Geometry: final body of the model. Coordinates: model frame, mm. Face numbers are marked on the shaded views. A direction names the side the tool comes from. Give positions to 0.01 mm unless a question says otherwise; leave off trailing zeros. Order: outer loops, then holes, each group sorted by start corner. A loop starts at its lowest first (then second) coordinate and runs counter-clockwise, first axis right, second up. Notation, with made-up numbers: (61, -24.75) - (98, -24.75) arc R20 cw to (98, -0.75) - close; hole circle Ø4 at (4.5, 2.25). An arc over 180 degrees is marked (long way). One line per item, written item: value.
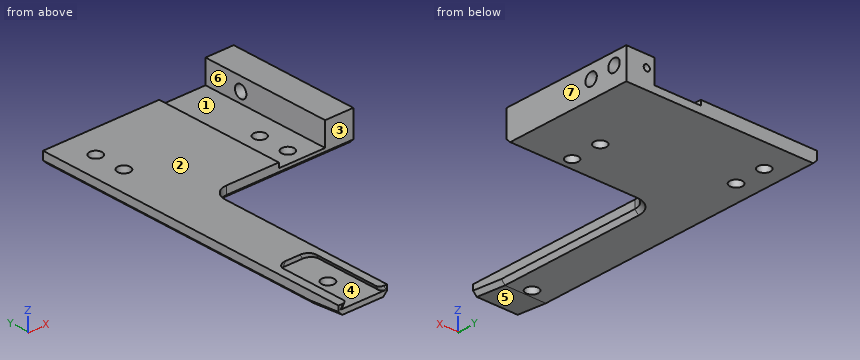
Autodesk Fusion 360 part; units mm, degrees
sketch "Sketch1" plane through (0, 0, 0) normal (0, 1, 0) x (1, 0, 0)
  line L0 (-12.4, 0.775) -> (12.4, 0.775)
  line L1 (12.4, 0.775) -> (12.4, -0.775)
  line L2 (12.4, -0.775) -> (-12.4, -0.775)
  line L3 (-12.4, -0.775) -> (-12.4, 0.775)
  line L4 (-12.4, 0.775) -> (12.4, -0.775) construction
  line L5 (12.4, 0.775) -> (-12.4, -0.775) construction
  dimension "d1" = 24.8
  dimension "d2" = 1.55
extrude "Extrude1" add sketch "Sketch1" along normal mid plane 17
sketch "Sketch4" plane through (0, 8.5, 0) normal (0, 1, 0) x (-1, 0, 0)
  line L0 (12.4, -0.775) -> (12.4, 0.775)
  line L1 (12.4, 0.775) -> (-12.4, 0.775)
  line L2 (-12.4, 0.775) -> (-12.4, -0.775)
  line L3 (-12.4, -0.775) -> (12.4, -0.775)
  line L4 (7.0918, 0.775) -> (6.7692, 0.2162)
  line L5 (6.7692, 0.2162) -> (11.6308, 0.2162)
  line L6 (11.6308, 0.2162) -> (11.3082, 0.775)
  point P0 (9.2, 0.2162)
  dimension "d11" = 60
  dimension "d12" = 60
  dimension "d13" = 4.2164
  dimension "d14" = 0.5588
  dimension "d47" = 3.2
extrude "Extrude3" cut sketch "Sketch4" against normal up to surface (17 mm away) contours L1 L4 L5 L6
sketch "Sketch2" plane through (0, 8.5, 0) normal (0, 1, 0) x (-1, 0, 0)
  line L0 (7.0918, 0.775) -> (-12.4, 0.775)
  line L1 (-12.4, 0.775) -> (-12.4, -0.775)
  line L2 (-12.4, -0.775) -> (12.4, -0.775)
  line L3 (12.4, -0.775) -> (12.4, 0.775)
  line L4 (-2.7118, 0.141) -> (-8.7318, 0.141)
  line L5 (-8.7318, 0.141) -> (-8.7318, 0.775)
  line L6 (-8.7318, 0.775) -> (-2.7118, 0.775)
  line L7 (-2.7118, 0.775) -> (-2.7118, 0.141)
  line L8 (6.7692, 0.2162) -> (7.0918, 0.775)
  line L9 (12.4, 0.775) -> (11.3082, 0.775)
  line L10 (11.3082, 0.775) -> (11.6308, 0.2162)
  line L11 (11.6308, 0.2162) -> (6.7692, 0.2162)
  dimension "d5" = 6.02
  dimension "d6" = 0.634
  dimension "d50" = 9.481
extrude "Extrude2" cut sketch "Sketch2" against normal up to surface (17 mm away) contours L0 L4 L5 L6 L7
sketch "Sketch6" plane through (0, 0, -0.775) normal (0, 0, -1) x (-1, 0, 0)
  line L0 (5.6836, 7) -> (5.6836, -7)
  line L1 (5.6836, -7) -> (6.75, -7)
  line L2 (6.75, -7) -> (6.75, 7)
  line L3 (6.75, 7) -> (5.6836, 7)
  line L4 (-0.15, 7) -> (-6.25, 7)
  line L5 (-5.7218, -6.5) -> (-5.7218, -2.5)
  line L6 (12.4, -8.5) -> (12.4, 8.5)
  line L7 (12.4, 8.5) -> (-12.4, 8.5)
  line L8 (-12.4, 8.5) -> (-12.4, -8.5)
  line L9 (-12.4, -8.5) -> (12.4, -8.5)
  curve L10
  line L11 (-2.7118, -8.5) -> (-8.7318, -8.5)
  line L12 (-8.7318, -8.5) -> (-8.7318, 8.5)
  line L13 (-8.7318, 8.5) -> (-2.7118, 8.5)
  line L14 (-2.7118, 8.5) -> (-2.7118, -8.5)
  point P0 (-5.7218, 7)
  point P1 (-5.7218, -2.5)
  point P2 (-5.7218, -6.5)
  point P3 (6.75, 0)
  point P4 (-5.7218, -4.5)
  point P5 (-5.7218, -8.5)
  point P6 (-5.7218, -8.5)
  dimension "d22" = 4
  dimension "d51" = 2
hole "Hole2" at (5.7218, -2.5, -0.775) at (5.7218, -6.5, -0.775) direction (0, 0, 1) diameter 1.6 depth 3.517 tip angle 118
sketch "Sketch7" plane through (0, 0, -0.775) normal (0, 0, -1) x (-1, 0, 0)
  line L0 (5.6836, 7) -> (5.6836, -7)
  line L1 (5.6836, -7) -> (6.75, -7)
  line L2 (6.75, -7) -> (6.75, 7)
  line L3 (6.75, 7) -> (5.6836, 7)
  line L4 (-6.25, -7) -> (-0.15, -7)
  circle A0 centre (-5.7218, -2.5) radius 0.8
  circle A1 centre (-5.7218, -6.5) radius 0.8
  line L5 (12.4, -8.5) -> (12.4, 8.5)
  line L6 (12.4, 8.5) -> (-12.4, 8.5)
  line L7 (-12.4, 8.5) -> (-12.4, -8.5)
  line L8 (-12.4, -8.5) -> (12.4, -8.5)
  point P0 (-3.2, -7)
  point P1 (-3.2, -4.5)
  dimension "d26" = 2.5
hole "Hole3" [suppressed]
extrude "Extrude4" add 1 faces at (11.1773, -2.8333, 0.775) along direction (0, 0, 1) blind 2.4
sketch "Sketch10" plane through (12.4, 0, 0) normal (1, 0, 0) x (0, 1, 0)
  line L0 (-8.5, -0.775) -> (8.5, -0.775)
  line L1 (8.5, -0.775) -> (8.5, 3.175)
  line L2 (8.5, 3.175) -> (-8.5, 3.175)
  line L3 (-8.5, 3.175) -> (-8.5, -0.775)
  point P0 (3.5, 1.475)
  dimension "d54" = 2.25
  dimension "d59" = 12
hole "Hole6" at (12.4, 3.5, 1.475) direction (-1, 0, 0) diameter 1.623 depth 6.5 tip angle 118
sketch "Sketch11" plane through (0, 8.5, 0) normal (0, 1, 0) x (-1, 0, 0)
  line L0 (11.6308, 0.2162) -> (6.7692, 0.2162)
  line L1 (7.0918, 0.775) -> (-2.7118, 0.775)
  line L2 (-2.7118, 0.775) -> (-2.7118, 0.141)
  line L3 (-2.7118, 0.141) -> (-8.7318, 0.141)
  line L4 (-8.7318, 0.141) -> (-8.7318, 3.175)
  line L5 (-8.7318, 3.175) -> (-12.4, 3.175)
  line L6 (-12.4, 3.175) -> (-12.4, -0.775)
  line L7 (-12.4, -0.775) -> (12.4, -0.775)
  line L8 (12.4, -0.775) -> (12.4, 0.775)
  line L9 (12.4, 0.775) -> (11.3082, 0.775)
  line L10 (11.3082, 0.775) -> (11.6308, 0.2162)
  line L11 (6.7692, 0.2162) -> (7.0918, 0.775)
  point P0 (-9.7318, 1.675)
  dimension "d60" = 1.5
  dimension "d61" = 1
hole "Hole7" at (9.7318, 8.5, 1.675) direction (0, -1, 0) diameter 0.8 depth 3 tip angle 118
sketch "Sketch12" plane through (12.4, 0, 0) normal (1, 0, 0) x (0, 1, 0)
  circle A0 centre (3.5, 1.475) radius 0.8115
  line L0 (-8.5, -0.775) -> (8.5, -0.775)
  line L1 (8.5, -0.775) -> (8.5, 3.175)
  line L2 (8.5, 3.175) -> (-8.5, 3.175)
  line L3 (-8.5, 3.175) -> (-8.5, -0.775)
  line L4 (8.5, 2.075) -> (8.5, 1.275)
  line L5 (5.5, 2.075) -> (5.5, 1.275)
  point P0 (6.75, 1.675)
  point P1 (8.5, 1.675)
  dimension "d66" = 1.75
hole "Hole8" at (12.4, 6.75, 1.675) direction (-1, 0, 0) diameter 1.623 depth 2.6 tip angle 118
fillet "Fillet1" [suppressed]
sketch "Sketch13" plane through (0, -8.5, 0) normal (0, -1, 0) x (1, 0, 0)
  line L0 (8.7318, 3.175) -> (8.7318, 0.141)
  line L1 (8.7318, 0.141) -> (2.7118, 0.141)
  line L2 (2.7118, 0.141) -> (2.7118, 0.775)
  line L3 (2.7118, 0.775) -> (-7.0918, 0.775)
  line L4 (-7.0918, 0.775) -> (-6.7692, 0.2162)
  line L5 (-6.7692, 0.2162) -> (-11.6308, 0.2162)
  line L6 (-11.6308, 0.2162) -> (-11.3082, 0.775)
  line L7 (-11.3082, 0.775) -> (-12.4, 0.775)
  line L8 (-12.4, 0.775) -> (-12.4, -0.775)
  line L9 (-12.4, -0.775) -> (12.4, -0.775)
  line L10 (12.4, -0.775) -> (12.4, 3.175)
  line L11 (12.4, 3.175) -> (8.7318, 3.175)
  line L12 (2.7118, 0.141) -> (2.7118, -0.775)
  line L13 (-6.0918, 0.775) -> (-6.0918, -0.775)
  dimension "d78" = 1
extrude "Extrude5" add sketch "Sketch13" along normal blind 25 contours L3 L4 L5 L6 L7 L8 L9 L13
sketch "Sketch5" plane through (0, 0, -0.775) normal (0, 0, -1) x (1, 0, 0)
  line L0 (-12.4, -8.5) -> (12.4, -8.5)
  line L1 (12.4, -8.5) -> (12.4, 8.5)
  line L2 (12.4, 8.5) -> (-6.0918, 8.5)
  line L3 (-12.4, 33.5) -> (-12.4, -8.5)
  circle A0 centre (5.7218, 2.5) radius 0.8
  circle A1 centre (5.7218, 6.5) radius 0.8
  line L4 (-6.0918, 33.5) -> (-12.4, 33.5)
  line L5 (-6.7692, 33.5) -> (-11.6308, 33.5)
  line L6 (-6.0918, 8.5) -> (-6.0918, 33.5)
  point P0 (-9.2, 33.5)
  point P1 (-9.2, 28.5)
  dimension "d72" = 5
hole "Hole1" at (-9.2, -28.5, -0.775) direction (0, 0, 1) diameter 1.623 end through all
sketch "Sketch14" plane through (-6.0918, 0, 0) normal (1, 0, 0) x (0, 1, 0)
  line L0 (-8.5, 0.243) -> (8.5, 0.243)
  line L1 (8.5, 0.243) -> (8.5, 0.875)
  line L2 (8.5, 0.875) -> (-8.5, 0.875)
  line L3 (-8.5, 0.875) -> (-8.5, 0.243)
  line L4 (-33.5, -0.425) -> (-29.5, -0.775)
  line L5 (-8.5, -0.775) -> (-8.5, 0.775)
  line L6 (-8.5, 0.775) -> (-33.5, 0.775)
  line L7 (-33.5, 0.775) -> (-33.5, -0.775)
  line L8 (-33.5, -0.775) -> (-8.5, -0.775)
  dimension "d88" = 4
  dimension "d89" = 0.35
extrude "Extrude6" cut sketch "Sketch14" against normal through all contours L4 L7 L8
fillet "Fillet2" radius 0.5 2 edges at (-11.4695, -33.5, 0.4956) (-6.9305, -33.5, 0.4956)
sketch "Sketch15" plane through (0, 8.5, 0) normal (0, 1, 0) x (-1, 0, 0)
  circle A0 centre (-9.7318, 1.675) radius 0.4
  line L0 (-8.7318, 0.141) -> (-8.7318, 3.175)
  line L1 (-8.7318, 3.175) -> (-12.4, 3.175)
  line L2 (-12.4, 3.175) -> (-12.4, -0.775)
  line L3 (-12.4, -0.775) -> (12.4, -0.775)
  line L4 (12.4, -0.775) -> (12.4, 0.775)
  line L5 (12.4, 0.775) -> (11.3082, 0.775)
  line L6 (11.3082, 0.775) -> (11.6308, 0.2162)
  line L7 (11.6308, 0.2162) -> (6.7692, 0.2162)
  line L8 (6.7692, 0.2162) -> (7.0918, 0.775)
  line L9 (7.0918, 0.775) -> (-2.7118, 0.775)
  line L10 (-2.7118, 0.775) -> (-2.7118, 0.141)
  line L11 (-2.7118, 0.141) -> (-8.7318, 0.141)
  line L12 (7.0918, 0.775) -> (11.3082, 0.775)
extrude "Extrude7" add sketch "Sketch15" against normal blind 32 contours L6 L7 L8 L12
sketch "Sketch16" plane through (0, 0, 0.775) normal (0, 0, 1) x (-1, 0, 0)
  ellipse E0 centre (11.8856, 33) end of major axis (11.3082, 33) minor radius 0.5 (11.8856, 33.5) -> (11.3082, 33) ccw
  line L0 (11.3082, 33) -> (11.3082, 23.5)
  line L1 (11.3082, 23.5) -> (7.0918, 23.5)
  line L2 (7.0918, 23.5) -> (7.0918, 33)
  ellipse E1 centre (6.5144, 33) end of major axis (7.0918, 33) minor radius 0.5 (7.0918, 33) -> (6.5144, 33.5) ccw
  line L3 (6.5144, 33.5) -> (6.0918, 33.5)
  line L4 (6.0918, 33.5) -> (6.0918, 8.5)
  line L5 (6.0918, 8.5) -> (-2.7118, 8.5)
  line L6 (-2.7118, 8.5) -> (-2.7118, -8.5)
  line L7 (-2.7118, -8.5) -> (12.4, -8.5)
  line L8 (12.4, -8.5) -> (12.4, 33.5)
  line L9 (12.4, 33.5) -> (11.8856, 33.5)
  point P0 (9.2, 23.5)
  point P1 (9.2, -4.5)
  point P2 (9.2, -0.5)
  dimension "d81" = 4
  dimension "d85" = 4
hole "Hole9" at (-9.2, 4.5, 0.775) at (-9.2, 0.5, 0.775) direction (0, 0, -1) diameter 1.623 depth 9 tip angle 118
fillet "Fillet3" radius 1 2 edges at (-6.9305, -23.5, 0.4956) (-11.4695, -23.5, 0.4956)
fillet "Fillet4" radius 2 1 edges at (-6.0918, -8.5, 0)
chamfer "Chamfer1" distance 0.5 angle 45 3 edges at (-6.0918, -31.5, -0.6) (-12.4, -31.5, -0.6) (-12.4, -10.5, -0.775)
equation "d6 = 0.75 mm - 0.116 mm"
1) Section D-D, the plane x = 3.25. Return loops of the section in (y, z) (3 decimals), then the cut area to 3 significant figures.
Answers below:
outline: (-8.5, -0.275) - (-8, -0.775) - (8.5, -0.775) - (8.5, 0.141) - (-8.5, 0.141) - close
area: 15.4 mm^2
2) Section C-C, the plane y = -25.5. Return loops of the section in (x, z) (3 decimals), then the cut area to 3 significant figures.
Answers below:
outline: (-12.4, -0.275) - (-11.9, -0.775) - (-6.592, -0.775) - (-6.092, -0.275) - (-6.092, 0.775) - (-7.092, 0.775) - (-6.769, 0.216) - (-11.631, 0.216) - (-11.308, 0.775) - (-12.4, 0.775) - close
area: 6.99 mm^2
3) First-contact query: pin 1 (1.9 mm diameter, centred on x = -9.2, y = 4.5, fed in from +Z) (3 decimals); pin 2 (1.5 mm diameter, centred on x = 5, y = -3.5, fed in from +Z); pin 3 (1.2 mm diameter, centred on y = -17, z = 0, fed in from +X). Flat tips, straight axial feed; report the tip coordinate or a pass-through.
Answers below:
pin 1: z = 0.775
pin 2: z = 0.14
pin 3: x = -6.09
4) Mould query, pull axis X, two halves, no side actions, for the marked faces 4, 5, 6 and 7. Classes: released by +X, released by -X, zero draft, split by the parting line, or undercut.
Answers below:
face 4: undercut
face 5: zero draft
face 6: undercut
face 7: released by +X
5) Set-up query: the marked faces 1, 2 and 3. Return all of +Z, -Z, +X, -X, +Y, -Y with unobstructed straight access to the full face (end or side cutting, diameter ignored); none if empty.
Answers below:
face 1: +Z, +Y, -Y
face 2: +Z, -X, +Y, -Y
face 3: +Z, -Z, +X, -Y
6) Section A-A, the plane y = 0.5. Return loops of the section in (x, z) (1 decimal).
Answers below:
outline: (-12.4, -0.3) - (-11.9, -0.8) - (-10, -0.8) - (-10, 0.8) - (-12.4, 0.8) - close; (-8.4, -0.8) - (12.4, -0.8) - (12.4, 3.2) - (8.7, 3.2) - (8.7, 0.1) - (2.7, 0.1) - (2.7, 0.8) - (-8.4, 0.8) - close
7) Material intervals for line 1 along Y through (x, z) = (-9.2, -0.3); line 2 along Y through (x, z) = (6.25, -0.1); line 3 along Z through (x, y) = (10.6, 6.75) (1 decimal), sorted ascending.
Answers below:
line 1: -33.5 to -29.31, -27.69 to -0.31, 1.31 to 3.69, 5.31 to 8.5
line 2: -8.5 to -7.1, -5.9 to -3.1, -1.9 to 8.5
line 3: -0.8 to 0.9, 2.5 to 3.2
8) Section B-B, the plane x = -9.2. Count the separate pieces of the cut face and the enclosed holes in it, then the cut area to 3 significant figures.
Answers below:
separate pieces: 4
enclosed holes: 0
area: 52.2 mm^2
